For this review, take the finished solid that the model builds, in its own axes (mm). A direction names the side the tool comes from. Give positions to 0.01 mm unless a question says otherwise; leave off trailing zeros. Write each loop counter-clockwise with the first axis right and the second up, starting at its lowest first coordinate (ties: lowest second). Pieces come first, ordered by that corner, then holes.
Q1. For line 1 (Z direction, x = 23, y = -33.5); line 2 (Z direction, x = 24, y = -124); line 3 (X direction, y = -12.5, z = -47), list the stretches that pass through material, from the lowest coordinate up.
Q2. We need section B-B (y = -62). Write out the cut boundary in (x, z).
Q3. Mouldability with a two-part tool opening along Z and no side actions: class faces 1 (the flat face through (64, -133.749, -5)), 2 (the conical face through (57.859, -112.274, -1.273)), 3 (the cylindrical face through (66.786, -13.748, 1.469)) as released by +Z, released by -Z, zero draft, split by the parting line, or undercut.
Q4. Machinability: for faces 4 (the cylindrical face through (73.134, -86.594, -1.609)), 5 (the cylindrical face through (60.437, -51.153, -1.329)), 6 (the flat face through (66.2, -38.1, 11.2)), which of the approach directions +Z, -Z, +X, -X, +Y, -Y give a long, thin tool a straight path to every point of the face, cutting with its end or side? Answer none if there is none.
Q5. Insertion check: P1, Ø12, axis at x = 19, y = -37, coming from the -Z side; P2, Ø2, axis at y = -21.5, z = -10.5, coming from the +X side; P3, Ø1, axis at y = -104, z = -24, coming from the -X side. Each pin has a flat end and moves straight along its axis. Give the tip position at first contact, or say it passes through.
Q6. We need section A-A (z = 0). Write out the cut boundary in (x, y), then the cut area to 3 significant figures.
Autodesk Inventor part; units mm, degrees
ref_plane "YZ Plane" through (0, 0, 0) normal (1, 0, 0) x (0, 1, 0)
ref_plane "XZ Plane" through (0, 0, 0) normal (0, 1, 0) x (-1, 0, 0)
ref_plane "XY Plane" through (0, 0, 0) normal (0, 0, 1) x (1, 0, 0)
sketch "Sketch1" plane through (0, 0, 0) normal (0, 0, 1) x (1, 0, 0)
  line L0 (0, 25.4) -> (-28.702, 25.4) construction
  line L1 (0, 25.4) -> (-86.36, 25.4) construction
  line L2 (-86.36, 25.4) -> (-80.01, 25.4) construction
  line L3 (-80.01, 25.4) -> (-73.66, 22.4389) construction
  line L4 (-80.01, 25.4) -> (-80.01, 22.4389) construction
  line L5 (-80.01, 0) -> (-86.36, 0)
  line L6 (-28.702, 59.6457) -> (-28.702, -91.9304) construction
  arc A0 (-28.9184, -4.2142) -> (-32.3684, 3.1843) centre (-35.052, -2.5707) ccw
  line L7 (-67.31, -147.4937) -> (-28.9184, -4.2142)
  line L8 (-80.01, 22.4389) -> (-73.66, 22.4389)
  line L9 (-80.01, 22.4389) -> (-80.01, 0)
  line L10 (-73.66, 22.4389) -> (-32.3684, 3.1843)
  line L11 (-28.702, -2.5707) -> (-60.452, -2.5707) construction
  line L12 (-60.452, 16.28) -> (-60.452, -121.8993) construction
  line L13 (-60.452, -121.8993) -> (-54.102, -121.8993) construction
  line L14 (-54.102, -121.8993) -> (-54.102, -98.2008) construction
  line L15 (-54.102, -98.2008) -> (-60.452, -98.2008)
  line L16 (-60.452, 16.28) -> (-60.452, 6.755) construction
  line L17 (-60.452, 16.28) -> (-60.452, 9.93) construction
  line L18 (-60.452, 9.93) -> (-46.8344, 9.93)
  line L19 (-60.452, 9.93) -> (-60.452, -98.2008)
  line L20 (-86.36, 0) -> (-86.36, -12.7) construction
  line L21 (-60.452, -12.7) -> (-73.152, -12.7) construction
  line L22 (-86.36, -12.7) -> (-86.36, -25.4) construction
  line L23 (-86.36, -25.4) -> (-86.36, -88.9) construction
  line L24 (-86.36, -88.9) -> (-73.66, -88.9) construction
  line L25 (-73.66, -88.9) -> (-73.66, -25.4) construction
  line L26 (-86.36, -25.4) -> (-73.66, -25.4)
  line L27 (-73.66, -25.4) -> (-73.66, -88.9)
  line L28 (-73.66, -88.9) -> (-86.36, -88.9)
  line L29 (-86.36, -12.7) -> (-73.152, -12.7)
  line L30 (-73.152, -133.7486) -> (-63.627, -133.7486)
  line L31 (-73.66, -88.9) -> (-73.66, -147.4937)
  line L32 (-73.66, -147.4937) -> (-67.31, -147.4937)
  line L33 (-73.152, -12.7) -> (-73.152, -133.7486)
  line L34 (-80.01, -25.4) -> (-80.01, -31.3436)
  line L35 (-80.01, -31.3436) -> (-86.36, -31.3436)
  line L36 (-86.36, 0) -> (-86.36, -25.4)
  line L37 (-86.36, -31.3436) -> (-86.36, -88.9)
  line L38 (0, -319.0244) -> (0, 122.7573)
  point P0 (0, 0)
  point P1 (-86.36, -255.9127)
  point P2 (-76.835, 22.4389)
  dimension "d0" = 28.702
  dimension "d1" = 86.36
  dimension "d2" = 6.35
  dimension "d3" = 25
  dimension "d5" = 25.4
  dimension "d6" = 25.4
  dimension "d8" = 12.7
  dimension "d11" = 6.35
  dimension "d12" = 31.75
  dimension "d13" = 6.35
  dimension "d15" = 6.35
  dimension "d16" = 12.7
  dimension "d17" = 12.7
  dimension "d18" = 12.7
  dimension "d19" = 63.5
  dimension "d20" = 12.7
  dimension "d22" = 9.525
  dimension "d23" = 6.35
  dimension "d25" = 5.9436
  dimension "d26" = 15
revolve "Revolution2" add sketch "Sketch1" angle 360 about axis through (0, -10, 0) along (0, 1, 0) contours L9 L8 L10 L18 L19 L15 L7 L30 L33 L29 L36 L5
sketch "Sketch2" plane through (0, 0, 0) normal (0, 1, 0) x (-1, 0, 0)
  line L0 (0, -114.5678) -> (107.9834, -114.5678)
  line L1 (107.9834, -114.5678) -> (107.9834, 108.3126)
  line L2 (107.9834, 108.3126) -> (0, 108.3126)
  line L3 (0, 108.3126) -> (0, -114.5678)
  point P0 (0, 0)
extrude "Extrusion1" cut sketch "Sketch2" along normal through all both and the other way through all
sketch "Sketch6" plane through (0, -133.7486, -73.152) normal (-1, 0, 0) x (0, 0, 1)
  line L0 (0, 121.0486) -> (0, 95.6486)
  line L1 (0, 95.6486) -> (6.35, 95.6486)
  line L2 (0, 121.0486) -> (-13.208, 121.0486)
  line L3 (-13.208, 121.0486) -> (-13.208, 133.7486)
  line L4 (-13.208, 121.0486) -> (-13.208, 133.7486)
  line L5 (-13.208, 133.7486) -> (-6.858, 133.7486)
  line L6 (-6.858, 133.7486) -> (-6.858, 156.1875)
  line L7 (-0.508, 156.1875) -> (26.3176, 143.6785)
  line L8 (-6.858, 156.1875) -> (-0.508, 156.1875)
  line L9 (-0.508, 156.1875) -> (26.3176, 143.6785)
  line L10 (6.35, 95.6486) -> (6.35, 143.68)
  line L11 (6.35, 143.68) -> (26.3176, 143.6785)
  line L12 (26.3176, 143.6785) -> (92.5608, 143.6785) construction
  line L13 (73.152, 133.7486) -> (73.152, 183.9478) construction
  line L14 (119.9864, 143.6785) -> (26.3176, 143.6785) construction
  line L15 (26.3176, 143.6785) -> (73.152, 143.6785) construction
  dimension "d37" = 25.4
  dimension "d38" = 6.35
  dimension "d39" = 6.35
  dimension "d40" = 48.0314
revolve "Revolution4" cut sketch "Sketch6" angle 360 about axis through (0, 0, 0) along (0, 1, 0)
sketch "Sketch7" plane through (0, 9.93, 0) normal (0, -1, 0) x (1, 0, 0)
  point P0 (0, 0)
sketch "Sketch8" plane through (0, 9.93, 0) normal (0, -1, 0) x (1, 0, 0)
  point P0 (0, 0)
sketch "Sketch9" plane through (0, 9.93, 0) normal (0, -1, 0) x (1, 0, 0)
  circle A0 centre (0, 0) radius 60.7129
extrude "Extrusion2" cut sketch "Sketch9" along normal mid plane 25.4
properties part number "part 1 phenolic sketch" material "Phenolic Resin"
Computed:
1. line 1: z = -62.72 to -55.91, 55.91 to 62.72
1. line 2: z = -69.1 to -56.1, 56.1 to 69.1
1. line 3: x = 38.02 to 47.47
2. outline: (0, -73.15) arc R73.15 ccw to (0, 73.15) - (0, 60.45) arc R60.45 cw to (0, -60.45) - close
3. face 1: zero draft
3. face 2: undercut
3. face 3: split by the parting line
4. face 4: +X, +Y, -Y
4. face 5: -X, +Y
4. face 6: +X, +Y
5. P1: stops at z = -71.97
5. P2: stops at x = 66.12
5. P3: stops at x = 49.93
6. outline: (54.1, -98.2) - (63.63, -133.75) - (73.15, -133.75) - (73.15, -38.1) - (66.8, -38.1) - (66.8, 9.93) - (60.71, 9.93) - (60.71, -2.77) - (60.45, -2.77) - (60.45, -98.2) - close
6. area: 1,570 mm2
